from build123d import *

# Parameters (mm, degrees)
CROQUIS1_R              = 4.5
CROQUIS1_R_2            = 2.55
SALIENTE_EXTRUIR1_DEPTH = 11
CROQUIS3_R              = 3.292391304
CROQUIS5_W              = 1.25
CROQUIS5_H              = 4.5


with BuildPart() as part:
    # Croquis1 → Saliente-Extruir1 (new body)
    with BuildSketch(Plane(origin=(0, 0, 0), x_dir=(1, 0, 0), z_dir=(0, 1, 0))):
        with Locations(Location((0, 0, 0), (0, 0, 270))):
            Circle(CROQUIS1_R)
        with Locations(Location((0, 0, 0), (0, 0, 270))):
            Circle(CROQUIS1_R_2, mode=Mode.SUBTRACT)
    extrude(amount=SALIENTE_EXTRUIR1_DEPTH)

    # Croquis3 → Cortar-Revolución1 (revolve, cut)
    with BuildSketch(Plane(origin=(0, 0, 0), x_dir=(0, 0, -1), z_dir=(1, 0, 0))):
        with Locations((-6.642391304, 7.5)):
            Circle(CROQUIS3_R)
    revolve(axis=Axis((0, 11, 0), (0, -1, 0)), mode=Mode.SUBTRACT)

    # Croquis5 → Taladro roscado M31 (revolve, cut)
    with BuildSketch(Plane(origin=(0, 2.5, 0), x_dir=(0, 1, 0), z_dir=(1, 0, 0))):
        with Locations((0.625, 2.25)):
            Rectangle(CROQUIS5_W, CROQUIS5_H)
    revolve(axis=Axis((0, 2.5, -6.35), (0, 0, 1)), mode=Mode.SUBTRACT)


solid = part.part
CAD build for the part. Positions are in the model's coordinates, mm. A direction names the side the tool comes from. Coordinates: 2 decimals unless noted, no trailing zeros. Loops run counter-clockwise (first coordinate to the right, second up) from the corner with the lowest first, then second, coordinate; pieces in that order, holes last. Notation, with made-up numbers: (24, 11) -> (32, 11) arc R18 cw to (32, 17) -> close; hole circle Ø4 at (84, 57). An arc over 180 degrees is marked (long way). One line per item, written item: value.
1. Pull direction X, two halves, no side cores. Call faces 3 (the face through (4.46, 2.47, -0.59)), 4 (the face through (-2, 11, 2)), 5 (the face through (0.112, 5.423, -2.548)): pulls with the +X half, pulls with the -X half, needs draft (parallel to the pull), parting line crosses it, or undercut.
Answers:
face 3: parting line crosses it
face 4: needs draft
face 5: undercut
2. Slice it at B-B on x = 0. Write the cut outline in (y, z), and give its area (3 significant figures).
Answers:
outline: (0, -4.5) -> (5, -4.5) arc R3.29 cw to (10, -4.5) -> (11, -4.5) -> (11, -2.55) -> (0, -2.55) -> close; (0, 2.55) -> (1.25, 2.55) -> (1.25, 4.5) -> (0, 4.5) -> close; (3.75, 2.55) -> (11, 2.55) -> (11, 4.5) -> (10, 4.5) arc R3.29 cw to (5, 4.5) -> (3.75, 4.5) -> close
area: 30.0 mm^2
3. Slice it at A-A on z = 0. Write the cut outline in (x, y), and give its area (3 significant figures).
Answers:
outline: (-4.5, 0) -> (-2.55, 0) -> (-2.55, 11) -> (-4.5, 11) -> (-4.5, 10) arc R3.29 cw to (-4.5, 5) -> close; (2.55, 0) -> (4.5, 0) -> (4.5, 5) arc R3.29 cw to (4.5, 10) -> (4.5, 11) -> (2.55, 11) -> close
area: 34.9 mm^2
4. Drill centre lines: line 1 (X direction, y = 4, z = 0); line 2 (Z direction, x = 2, y = 5.5); line 3 (X direction, y = 8.25, z = 0). Where is each one in solid material? Low to high. Write a range as [from, to].
Answers:
line 1: x = [-4.5, -2.55], [2.55, 4.5]
line 2: z = [-3.5, -1.58], [1.58, 3.5]
line 3: x = [-3.44, -2.55], [2.55, 3.44]
5. Slice it at C-C on y = 4.75. Write the cut outline in (x, z), and give its area (3 significant figures).
Answers:
outline: circle Ø9 at (0, 0); hole circle Ø5.1 at (0, 0)
area: 43.2 mm^2
6. Flat gauge pins, fed straight in: P1, Ø2, axis at x = -3, z = 0.5, coming from the -Y side; P2, Ø1.5, axis at y = 6, z = 3.5, coming from the +X side. Where does each tip first touch, or does it go through?
Answers:
P1: stops at y = 0
P2: stops at x = 2.76
7. Slice it at D-D on y = 6.75. Write the cut outline in (x, z).
Answers:
outline: circle Ø6.87 at (0, 0); hole circle Ø5.1 at (0, 0)
8. Which spindle directions (+Z, -Z, +X, -X, +Y, -Y) get a long thin tool onto all of the face, cutting with end or side? Do faces 1 (the face through (-2, 0, 2)), 2 (the face through (-0.38, 3.69, 3.38)). Say none if no direction does.
Answers:
face 1: +Z, -Z, +X, -X, -Y
face 2: +Z
